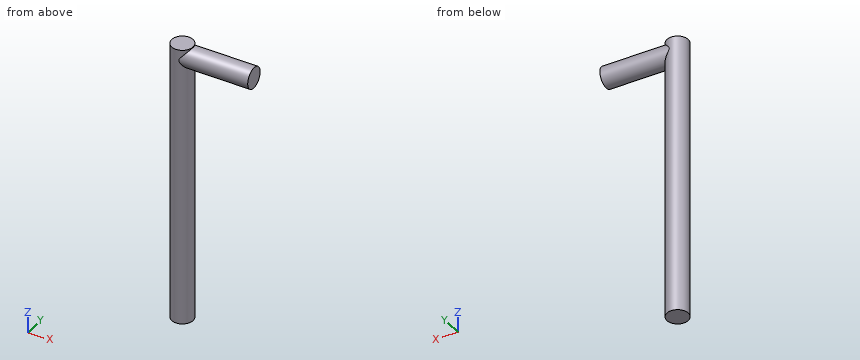
```python
from build123d import *

# Parameters (mm, degrees)
SKETCH3_R           = 1.5
BOSS_EXTRUDE1_DEPTH = 40
SKETCH4_W           = 10
SKETCH4_H           = 1.987336218
EXTRUDE_THIN1_DEPTH = 10
SKETCH7_R           = 1.464965711
BOSS_EXTRUDE4_DEPTH = 10
SKETCH9_W           = 11.25222939
SKETCH9_H           = 3.128852859
CUT_EXTRUDE1_DEPTH  = 57.344455031


with BuildPart() as part:
    # Sketch3 → Boss-Extrude1 (new body)
    with BuildSketch(Plane.XY):
        with Locations((-77.047665821, 20.487229207)):
            Circle(SKETCH3_R)
    extrude(amount=BOSS_EXTRUDE1_DEPTH)

    # Sketch4 → Extrude-Thin1 (add)
    with BuildSketch(Plane.XY.offset(40)):
        with Locations((-72.119350757, 22.979183427)):
            Rectangle(SKETCH4_W, SKETCH4_H)
    extrude(amount=EXTRUDE_THIN1_DEPTH)

    # Sketch7 → Boss-Extrude4 (add)
    with BuildSketch(Plane.ZY.offset(77.119350757)):
        with Locations((38.46487538, 20.493738907)):
            Circle(SKETCH7_R)
    extrude(amount=-BOSS_EXTRUDE4_DEPTH)

    # Sketch9 → Cut-Extrude1 (cut, through all)
    with BuildSketch(Plane.ZY.offset(77.119350757)):
        with Locations((45.626114695, 22.408425107)):
            Rectangle(SKETCH9_W, SKETCH9_H)
    extrude(amount=-CUT_EXTRUDE1_DEPTH, mode=Mode.SUBTRACT)


solid = part.part
```
Here's how the part is built. I have some questions about the finished solid (model axes, mm). Give positions to 0.01 mm unless a question says otherwise; leave off trailing zeros. Write each loop counter-clockwise with the first axis right and the second up, starting at its lowest first coordinate (ties: lowest second). Pieces come first, ordered by that corner, then holes.
(1) Imagine slicing it at B-B, the plane x = -76. Write out the boundary of the cut face in (y, z), and give its area (3 significant figures).
Output values:
outline: (19.41, 0) - (21.56, 0) - (21.56, 37.46) arc R1.46 ccw to (21.56, 39.47) - (21.56, 40) - (19.41, 40) - (19.41, 39.45) arc R1.46 ccw to (19.41, 37.48) - close
area: 87.0 mm2
(2) If I drill on L1, parallel to Z at x = -72.5, y = 20.6; L2, parallel to X at y = 20.1, z = 21; L3, parallel to Z at x = -71, y = 20.9, over which ranges is the centre line in solid material (lowest first)?
Output values:
L1: z = 37 to 39.93
L2: x = -78.5 to -75.6
L3: z = 37.06 to 39.87
(3) Imagine slicing it at C-C, the plane z = 26. Write out the boundary of the cut face in (x, y).
Output values:
outline: circle Ø3 at (-77.05, 20.49)
(4) Imagine slicing it at D-D, the plane x = -70.5. Write out the boundary of the cut face in (y, z), and give its area (3 significant figures).
Output values:
outline: circle Ø2.93 at (20.49, 38.46)
area: 6.74 mm2
(5) Imagine slicing it at A-A, the plane y = 19.55. Write out the boundary of the cut face in (x, z), and give its area (3 significant figures).
Output values:
outline: (-78.22, 0) - (-75.88, 0) - (-75.88, 37.34) - (-67.12, 37.34) - (-67.12, 39.59) - (-75.88, 39.59) - (-75.88, 40) - (-78.22, 40) - close
area: 113 mm2
(6) Will these pins go through, and if not, where does the flat tip stop? pin 1 (3 mm diameter, centred on x = -74.5, z = 19.5, fed in from -Y); pin 2 (1.5 mm diameter, centred on y = 21, z = 28, fed in from +X).
Output values:
pin 1: stops at y = 19.41
pin 2: stops at x = -75.55
